from build123d import *

# Parameters (mm, degrees)
SKETCH1_W           = 30
SKETCH1_H           = 30
SKETCH1_W_2         = 20
SKETCH1_H_2         = 20
BOSS_EXTRUDE1_DEPTH = 250
SKETCH2_W           = 30
SKETCH2_H           = 30
SKETCH2_R           = 2.5
BOSS_EXTRUDE2_DEPTH = 5


with BuildPart() as part:
    # Sketch1 → Boss-Extrude1 (new body)
    with BuildSketch(Plane(origin=(0, 0, 0), x_dir=(1, 0, 0), z_dir=(0, 1, 0))):
        with Locations((15, 15)):
            Rectangle(SKETCH1_W, SKETCH1_H)
        with Locations((15, 15)):
            Rectangle(SKETCH1_W_2, SKETCH1_H_2, mode=Mode.SUBTRACT)
    extrude(amount=BOSS_EXTRUDE1_DEPTH)

    # Sketch2 → Boss-Extrude2 (add)
    with BuildSketch(Plane(origin=(0, 250, 0), x_dir=(1, 0, 0), z_dir=(0, 1, 0))):
        with Locations((15, 15)):
            Rectangle(SKETCH2_W, SKETCH2_H)
        with Locations((15, 15)):
            Circle(SKETCH2_R, mode=Mode.SUBTRACT)
    extrude(amount=BOSS_EXTRUDE2_DEPTH)


solid = part.part
For this review, take the finished solid that the model builds, in its own axes (mm). A direction names the side the tool comes from. Give positions to 0.01 mm unless a question says otherwise; leave off trailing zeros. Order: outer loops, then holes, each group sorted by start corner. A loop starts at its lowest first (then second) coordinate and runs counter-clockwise, first axis right, second up. Notation, with made-up numbers: M 41,-35.5 L 60,-35.5 A20 cw 60,-28.5 Z; hole C 25.5,-10.5 d3. An arc over 180 degrees is marked long. Answer in a Markdown table with one row per item. Add a question column.
(1) For pin 1 (6 mm diameter, centred on x = 15, z = -15, fed in from -Y), flat-tipped, find the tip position at first contact; note if it passes through.
(2) For faces 4 (the face through (4.8, 0, -15.2)), 5 (the face through (13, 250, -13)), list the 3-axis set-ups (+Z, -Z, +X, -X, +Y, -Y) from which the entire face can be reached by the end or side of a thin tool; tool diameter is ignored.
(3) Consider section A-A on z = -15. State the section outline as (x, y) points.
(4) Consider section C-C on y = 148.5. State the section outline as (x, z) points, and give its area (3 significant figures).
(5) Mouldability with a two-part tool opening along Z and no side actions: class faces 1 (the face through (15, 126, 0)), 2 (the face through (25, 123, -15)), 3 (the face through (0, 126, -15)) as +Z half, -Z half, draft (parallel to the pull), parting line (faces both ways), or undercut.
(6) Wall thickness on probe 1 along X at (y, z) = (253.55, -15); probe 2 along Z at (x, y) = (9.75, 238); probe 3 along Z at (x, y) = (15, 253.7): over which ranges is each line inside the solid? List them lowest first. Write a range as [from, to].
(7) Consider section B-B on x = 15. State the section outline as (y, z) points.
Evaluation:
| question | item | result |
|---|---|---|
| 1 | pin 1 | stops at y = 250 |
| 2 | face 4 | +Z, -Z, +X, -X, -Y |
| 2 | face 5 | -Y |
| 3 | outline | M 0,0 L 5,0 L 5,250 L 12.5,250 L 12.5,255 L 0,255 Z; M 17.5,250 L 25,250 L 25,0 L 30,0 L 30,255 L 17.5,255 Z |
| 4 | outline | M 0,-30 L 30,-30 L 30,0 L 0,0 Z; hole M 5,-25 L 25,-25 L 25,-5 L 5,-5 Z |
| 4 | area | 500 mm^2 |
| 5 | face 1 | +Z half |
| 5 | face 2 | undercut |
| 5 | face 3 | draft |
| 6 | probe 1 | x = [0, 12.5], [17.5, 30] |
| 6 | probe 2 | z = [-30, -25], [-5, 0] |
| 6 | probe 3 | z = [-30, -17.5], [-12.5, 0] |
| 7 | outline | M 0,-30 L 255,-30 L 255,-17.5 L 250,-17.5 L 250,-25 L 0,-25 Z; M 0,-5 L 250,-5 L 250,-12.5 L 255,-12.5 L 255,0 L 0,0 Z |
